For this review, take the finished solid that the model builds, in its own axes (mm). Face numbers are marked on the shaded views. A direction names the side the tool comes from. Give positions to 0.01 mm unless a question says otherwise; leave off trailing zeros. Write each loop counter-clockwise with the first axis right and the second up, starting at its lowest first coordinate (ties: lowest second). Pieces come first, ordered by that corner, then holes.
Q1. We need section C-C (y = 4.5). Give the number of separate pieces and of enclosed holes in the cut face, then the cut area to 3 significant figures.
Q2. For line 1 (Z direction, x = -15, y = 1.75); line 2 (X direction, y = 2.45, z = 2.5); line 3 (Y direction, x = -32.5, z = 14) (3 decimals), list the stretches that pass through material, from the lowest coordinate up.
Q3. Mouldability with a two-part tool opening along Z and no side actions: class the marked faces 1, 2, 3 and 4 as released by +Z, released by -Z, zero draft, split by the parting line, or undercut.
Q4. We need section D-D (y = 7). Write out the cut boundary in (x, z).
Q5. Machinability: for the marked faces 5 and 6, which of the approach directions +Z, -Z, +X, -X, +Y, -Y give a long, thin tool a straight path to every point of the face, cutting with its end or side? Answer none if there is none.
Q6. We need section B-B (x = -30.5). Write out the cut boundary in (y, z) (3 decimals), then the cut area to 3 significant figures.
Q7. Insertion check: P1, Ø1.3, axis at x = 0.5, y = 8, coming from the +Z side; P2, Ø1.6, axis at x = -18.375, z = 2.5, coming from the -Y side; P3, Ø8, axis at y = 12, z = 6, coming from the +X side; P4, Ø6.5, axis at y = 13, z = 10, coming from the +X side. Each pin has a flat end and moves straight along its axis. Give the tip position at first contact, or say it passes through.
```python
from build123d import *

# Parameters (mm, degrees)
WALL_DEPTH                = 19.05
ROOF_START                = 19.05
ROOF_DEPTH                = 3.175
F_2_56_TAPPED_HOLE1_D     = 1.778
F_2_56_TAPPED_HOLE1_DEPTH = 5.73
F_2_56_TAPPED_HOLE1_TIP   = 0.53416509
BOSS_EXTRUDE1_DEPTH       = 1.5875
CUT_EXTRUDE3_DEPTH        = 2
FILLET1_R                 = 1.5875


with BuildPart() as part:
    # MainSketch → Wall (new body)
    with BuildSketch(Plane(origin=(0, 0, 0), x_dir=(1, 0, 0), z_dir=(0, 1, 0))):
        Polygon((-32.75, -4), (0, -4), (0, 0), (-36.75, 0), (-36.75, -45.5), (0, -45.5), (0, -41.5), (-32.75, -41.5), align=None)
    extrude(amount=WALL_DEPTH)

    # MainSketch<3> → Roof (add)
    with BuildSketch(Plane(origin=(0, 0, 0), x_dir=(1, 0, 0), z_dir=(0, 1, 0)).offset(ROOF_START)):
        with BuildLine():
            Line((0, -21.625), (0, 0))
            Line((0, 0), (-36.75, 0))
            Line((-36.75, 0), (-36.75, -45.5))
            Line((-36.75, -45.5), (0, -45.5))
            Line((0, -45.5), (0, -23.875))
            ThreePointArc((0, -23.875), (-0.353553391, -23.728553391), (-0.5, -23.375))
            Line((-0.5, -23.375), (-0.5, -22.125))
            ThreePointArc((-0.5, -22.125), (-0.353553391, -21.771446609), (0, -21.625))
        make_face()
    extrude(amount=ROOF_DEPTH)

    # #2-56 Tapped Hole1
    with Locations(Plane(origin=(-18.375, 0, 43), x_dir=(0, 0, -1), z_dir=(0, -1, 0))):
        with Locations((0, 0), (40.5, 0)):
            Hole(F_2_56_TAPPED_HOLE1_D / 2, depth=F_2_56_TAPPED_HOLE1_DEPTH)
            with Locations((0, 0, -(F_2_56_TAPPED_HOLE1_DEPTH + F_2_56_TAPPED_HOLE1_TIP / 2))):  # 118° drill point
                Cone(0, F_2_56_TAPPED_HOLE1_D / 2, F_2_56_TAPPED_HOLE1_TIP, mode=Mode.SUBTRACT)

    # Sketch3 → Boss-Extrude1 (add)
    with BuildSketch(Plane(origin=(0, 0, 0), x_dir=(0, 0, -1), z_dir=(1, 0, 0))):
        Polygon((-24.875, 21.1375), (-24.875, 20.1375), (-43, 20.1375), (-43, 0), (-44, 0), (-44, 21.1375), align=None)
    extrude(amount=BOSS_EXTRUDE1_DEPTH)

    # Sketch3<3> → Cut-Extrude3 (cut)
    with BuildSketch(Plane(origin=(0, 0, 0), x_dir=(0, 0, -1), z_dir=(1, 0, 0))):
        Polygon((-21.125, 19.8875), (-21.125, 21.3875), (-1.25, 21.3875), (-1.25, 0), (-2.75, 0), (-2.75, 19.8875), align=None)
    extrude(amount=-CUT_EXTRUDE3_DEPTH, mode=Mode.SUBTRACT)

    # Fillet1
    fillet1_edges = [part.edges().sort_by_distance(p)[0] for p in [
        (0.79375, 20.1375, 43),
        (0.79375, 21.1375, 44),
        (1.5875, 20.6375, 24.875),
        (-1, 21.3875, 1.25),
        (-1, 19.8875, 2.75),
        (-2, 20.6375, 21.125),
    ]]
    fillet(fillet1_edges, radius=FILLET1_R - 0.0001)  # a hair under: the kernel refuses the full size


solid = part.part
```
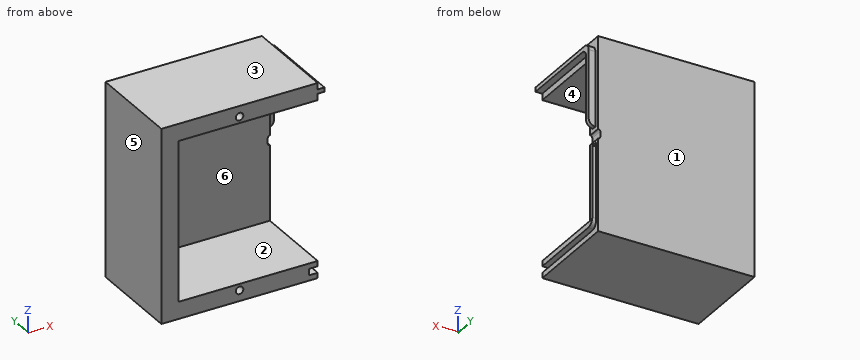
Computed:
1. separate pieces: 1
1. enclosed holes: 2
1. area: 438 mm2
2. line 1: z = 0 to 4, 41.5 to 45.5
2. line 2: x = -36.75 to -19.26, -17.49 to -2
2. line 3: y = 19.05 to 22.225
3. face 1: zero draft
3. face 2: undercut
3. face 3: released by +Z
3. face 4: undercut
4. outline: (-36.75, 0) - (0, 0) - (0, 1.25) - (-2, 1.25) - (-2, 2.75) - (0, 2.75) - (0, 4) - (-32.75, 4) - (-32.75, 41.5) - (0, 41.5) - (0, 43) - (1.59, 43) - (1.59, 44) - (0, 44) - (0, 45.5) - (-36.75, 45.5) - close
5. face 5: +Z, -Z, -X, +Y, -Y
5. face 6: +X, -Y
6. outline: (0, 0) - (22.225, 0) - (22.225, 45.5) - (0, 45.5) - (0, 41.5) - (19.05, 41.5) - (19.05, 4) - (0, 4) - close
6. area: 297 mm2
7. P1: stops at z = 45.5
7. P2: stops at y = 5.78
7. P3: stops at x = 0
7. P4: stops at x = -32.75
